from build123d import *

# Parameters (mm, degrees)
SKETCH1_R           = 152.4
BOSS_EXTRUDE1_DEPTH = 3.175
CUT_EXTRUDE2_START  = -3.175
SKETCH2_W           = 117.669510625
SKETCH2_H           = 6.35
CUT_EXTRUDE2_DEPTH  = 0.396875


with BuildPart() as part:
    # Sketch1 → Boss-Extrude1 (new body)
    with BuildSketch(Plane.XY):
        Circle(SKETCH1_R)
    extrude(amount=BOSS_EXTRUDE1_DEPTH)

    # Sketch2 → Cut-Extrude2 (cut)
    with BuildSketch(Plane(origin=(0, 0, 0), x_dir=(-1, 0, 0), z_dir=(0, 0, -1)).offset(CUT_EXTRUDE2_START)):
        with Locations((58.834755313, -146.05)):
            Rectangle(SKETCH2_W, SKETCH2_H)
    extrude(amount=CUT_EXTRUDE2_DEPTH, mode=Mode.SUBTRACT)


solid = part.part
Geometry check sheet. Reference: the model listing, model coordinates, mm. Round coordinates to 2 decimals unless told otherwise and drop trailing zeros. Order: outer loops, then holes, each group sorted by start corner. A loop starts at its lowest first (then second) coordinate and runs counter-clockwise, first axis right, second up. Notation, with made-up numbers: M -25.5,-40 L 22.5,-40 A20 ccw 22.5,-30 Z; hole C 31.5,-19 d5. An arc over 180 degrees is marked long. Answer in a Markdown table with one row per item.
(1) Scan lines: probe 1 along Y at (x, z) = (-4, 1.35); probe 2 along X at (y, z) = (115.5, 0.3); probe 3 along X at (y, z) = (-38.5, 0.7). Record each from-to range of solid material in increasing order. Write a range as from..to.
Responses:
| item | result |
|---|---|
| probe 1 | y = -152.35..152.35 |
| probe 2 | x = -99.43..99.43 |
| probe 3 | x = -147.46..147.46 |
(2) Sectioned sample at C-C, the plane y = 98. Record the cut outline in (x, z) (3 decimals), and give its area (3 significant figures).
Responses:
| item | result |
|---|---|
| outline | M -116.712,0 L 116.712,0 L 116.712,3.175 L -116.712,3.175 Z |
| area | 741 mm² |
(3) Go/stop test with flat-tipped pins: P1, Ø1, axis at x = -45.5, z = 2.5, coming from the -Y side; P2, Ø5, axis at x = -13.5, y = -146, coming from the +Z side. Record where each tip stops, or that it passes through.
Responses:
| item | result |
|---|---|
| P1 | stops at y = -145.6 |
| P2 | stops at z = 2.78 |
(4) Sectioned sample at B-B, the plane x = -65. Record the cut outline in (y, z) (3 decimals).
Responses:
| item | result |
|---|---|
| outline | M -137.843,0 L 137.843,0 L 137.843,3.175 L -137.843,3.175 Z |
(5) Sectioned sample at A-A, the plane z = 2.2. Record the cut outline in (x, y).
Responses:
| item | result |
|---|---|
| outline | C 0,0 d304.8 |
